```python
from build123d import *

# Parameters (mm, degrees)
F0_W        = 43.18
F0_H        = 6.35
F1_DEPTH    = 2.54
F2_T1_DEPTH = 27.94
F4_DEPTH    = 2.541


# Not quite as in the source:
# - a fillet or chamfer that OpenCascade refuses, or shapes differently, is made with other operations: its cross-section is extruded or revolved along the edge and cut away or added


with BuildPart() as f1:
    # F0 (on Top) → F1 (new body)
    with BuildSketch(Plane.XY):
        Rectangle(F0_W, F0_H)
    extrude(amount=F1_DEPTH)

    # F2: fillet of radius 5.08 on 4 edges, made by hand

    # F2_s2 → F2_t1 (cut)
    with BuildSketch(Plane.XY.offset(-12.7)):
        with BuildLine():
            ThreePointArc((21.59, 1.905), (20.1021024484, -1.6871024484), (16.51, -3.175))
            Line((16.51, -3.175), (21.59, -3.175))
            Line((21.59, -3.175), (21.59, 1.905))
        make_face()
        with BuildLine():
            ThreePointArc((21.59, -1.905), (20.1021024484, 1.6871024484), (16.51, 3.175))
            Line((16.51, 3.175), (21.59, 3.175))
            Line((21.59, 3.175), (21.59, -1.905))
        make_face()
        with BuildLine():
            ThreePointArc((-16.51, 3.175), (-20.1021024484, 1.6871024484), (-21.59, -1.905))
            Line((-21.59, -1.905), (-21.59, 3.175))
            Line((-21.59, 3.175), (-16.51, 3.175))
        make_face()
        with BuildLine():
            ThreePointArc((-21.59, 1.905), (-20.1021024484, -1.6871024484), (-16.51, -3.175))
            Line((-16.51, -3.175), (-21.59, -3.175))
            Line((-21.59, -3.175), (-21.59, 1.905))
        make_face()
    extrude(amount=F2_T1_DEPTH, mode=Mode.SUBTRACT)

    # F3 (on face) → F4 (cut, through all)
    with BuildSketch(Plane.XY.offset(2.54)):
        with BuildLine():
            Line((15.1645667607, 0), (19.3645667607, 0))
            ThreePointArc((19.3645667607, 0), (17.2645667607, 2.1), (15.1645667607, 0))
        make_face()
        with BuildLine():
            ThreePointArc((-9.7229412393, -2.1), (-8.2380169988, -1.4849242405), (-7.6229412393, 0))
            Line((-7.6229412393, 0), (-18.2392860393, 0))
            ThreePointArc((-18.2392860393, 0), (-17.6242102798, -1.4849242405), (-16.1392860393, -2.1))
            Line((-16.1392860393, -2.1), (-9.7229412393, -2.1))
        make_face()
        with BuildLine():
            Line((-18.2392860393, 0), (-7.6229412393, 0))
            ThreePointArc((-7.6229412393, 0), (-8.2380169988, 1.4849242405), (-9.7229412393, 2.1))
            Line((-9.7229412393, 2.1), (-16.1392860393, 2.1))
            ThreePointArc((-16.1392860393, 2.1), (-17.6242102798, 1.4849242405), (-18.2392860393, 0))
        make_face()
        with BuildLine():
            ThreePointArc((-6.4254332393, 0), (-4.3254332393, -2.1), (-2.2254332393, 0))
            Line((-2.2254332393, 0), (-6.4254332393, 0))
        make_face()
        with BuildLine():
            Line((-6.4254332393, 0), (-2.2254332393, 0))
            ThreePointArc((-2.2254332393, 0), (-4.3254332393, 2.1), (-6.4254332393, 0))
        make_face()
        with BuildLine():
            ThreePointArc((15.1645667607, 0), (17.2645667607, -2.1), (19.3645667607, 0))
            Line((19.3645667607, 0), (15.1645667607, 0))
        make_face()
    extrude(amount=-F4_DEPTH, mode=Mode.SUBTRACT)


solid = f1.part
```
Work out the finished part from the listing and answer in its coordinate system (mm). A direction names the side the tool comes from. Give positions to 0.01 mm unless a question says otherwise; leave off trailing zeros. Write each loop counter-clockwise with the first axis right and the second up, starting at its lowest first coordinate (ties: lowest second). Pieces come first, ordered by that corner, then holes. Notation, with made-up numbers: (64.25, -24.75) -> (118.25, -24.75) arc R28 ccw to (118.25, 14.25) -> close; hole circle Ø2 at (64, 55). An arc over 180 degrees is marked (long way). Write item = value, one per line.
Q1. Section B-B on z = 0.5 is taken. Determine the outline of the cut face in (x, y) (3 decimals), and give its area (3 significant figures).
Computed values:
outline = (-21.219, 0) arc R5.08 ccw to (-16.51, -3.175) -> (16.51, -3.175) arc R5.08 ccw to (21.219, 0) arc R5.08 ccw to (16.51, 3.175) -> (-16.51, 3.175) arc R5.08 ccw to start; hole (-16.139, -2.1) -> (-9.723, -2.1) arc R2.1 ccw to (-9.723, 2.1) -> (-16.139, 2.1) arc R2.1 ccw to start; hole circle Ø4.2 at (-4.325, 0); hole circle Ø4.2 at (17.265, 0)
area = 184 mm^2
Q2. Section C-C on x = -6 is taken. Determine the outline of the cut face in (y, z) (3 decimals).
Computed values:
outline = (-3.175, 0) -> (-1.267, 0) -> (-1.267, 2.54) -> (-3.175, 2.54) -> close; (1.267, 0) -> (3.175, 0) -> (3.175, 2.54) -> (1.267, 2.54) -> close
Q3. Section A-A on x = -12.5 is taken. Determine the outline of the cut face in (y, z) (3 decimals), and give its area (3 significant figures).
Computed values:
outline = (-3.175, 0) -> (-2.1, 0) -> (-2.1, 2.54) -> (-3.175, 2.54) -> close; (2.1, 0) -> (3.175, 0) -> (3.175, 2.54) -> (2.1, 2.54) -> close
area = 5.46 mm^2
Q4. Consider line 1 along X through (y, z) = (-0.25, 1.75); line 2 along X through (y, z) = (0.5, 0.3); line 3 along Y through (x, z) = (-11, 1.4) (3 decimals). Determine where each line is inside the solid, lowest interval first.
Computed values:
line_1 = -21.11 to -18.22, -7.64 to -6.41, -2.24 to 15.18, 19.35 to 21.11
line_2 = -20.98 to -18.18, -7.68 to -6.37, -2.29 to 15.22, 19.3 to 20.98
line_3 = -3.175 to -2.1, 2.1 to 3.175
Q5. For a pull along Y with two mould halves and no side action, classify faces 1 (the flat face through (0, 3.175, 1)), 2 (the cylindrical face through (19.363, -0.092, 1.288)), 3 (the cylindrical face through (19.385, -2.283, 1.252)) as pulls with the +Y half, pulls with the -Y half, needs draft (parallel to the pull), parting line crosses it, or undercut.
Computed values:
face_1 = pulls with the +Y half
face_2 = undercut
face_3 = pulls with the -Y half
Q6. A tool of negligible diameter and unlimited length cuts with its end or side. For faces 4 (the flat face through (-13, 2.1, 1)), 5 (the flat face through (0, 0, 2.54)), from which of +Z, -Z, +X, -X, +Y, -Y can it reach the whole face along a straight path? Write none if from no direction.
Computed values:
face_4 = +Z, -Z
face_5 = +Z, +X, -X, +Y, -Y
